Job drawing, mm, ordinate dimensions from the low corner. One solid piece. Round coordinates to 2 decimals unless told otherwise and drop trailing zeros. Order: outer loops, then holes, each group sorted by start corner. A loop starts at its lowest first (then second) coordinate and runs counter-clockwise, first axis right, second up. Notation, with made-up numbers: M 11,78.5 L 64,78.5 A17 cw 64,96.5 Z; hole C 52.5,53 d11. An arc over 180 degrees is marked long. Answer as a JSON object with one key per item and string values. Group by question number.
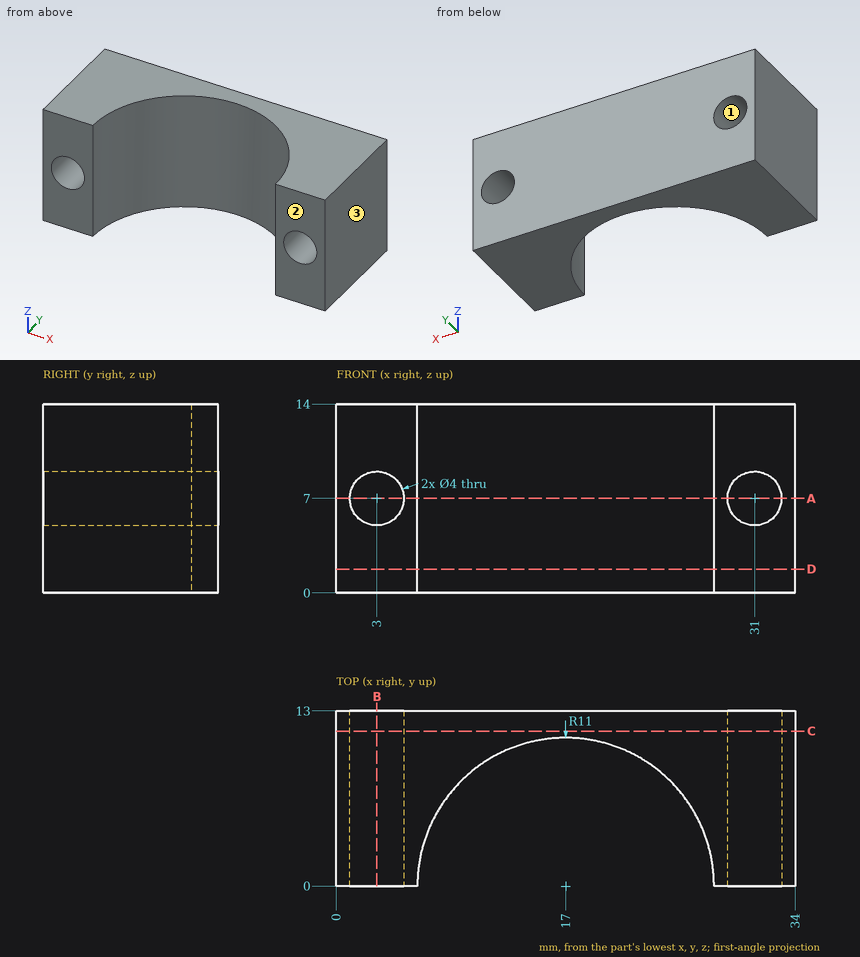
Item 1: Cut at B-B, the plane x = 3. Give the cut face in (y, z), and give its area (3 significant figures).
Item 2: Cut at C-C, the plane y = 11.5. Give the cut face in (x, z), and give its area (3 significant figures).
Item 3: Flat gauge pin, fed straight in: pin 1 Ø1 at (x, z) = (14.5, 12) entering from -Y. Where does the tip first touch, or does it go through?
Item 4: Drill centre lines: line 1 (Z direction, x = 3, y = 2.5); line 2 (X direction, y = 3, z = 7); line 3 (X direction, y = 9, z = 5.5). Where is each one in solid material? Low to high. Write a range as [from, to].
Item 5: Cut at D-D, the plane z = 1.75. Give the cut face in (x, y).
Item 6: Two-plate mould, pull along X, no slides. Class the marked faces 1, 2 and 3: +X half, -X half, draft (parallel to the pull), parting line (faces both ways), or undercut.
Item 7: Cut at A-A, the plane z = 7. Give the cut face in (x, y), and give its area (3 significant figures).
Response values:
{
 "1": {"outline": "M 0,0 L 13,0 L 13,5 L 0,5 Z; M 0,9 L 13,9 L 13,14 L 0,14 Z", "area": "130 mm^2"},
 "2": {"outline": "M 0,0 L 34,0 L 34,14 L 0,14 Z; hole C 3,7 d4; hole C 31,7 d4", "area": "451 mm^2"},
 "3": {"pin 1": "y = 10.58"},
 "4": {"line 1": "[0, 5], [9, 14]", "line 2": "[0, 1], [5, 6.42], [27.58, 29], [33, 34]", "line 3": "[0, 1.68], [4.32, 10.68], [23.32, 29.68], [32.32, 34]"},
 "5": {"outline": "M 0,0 L 6,0 A11 cw 28,0 L 34,0 L 34,13 L 0,13 Z"},
 "6": {"face 1": "undercut", "face 2": "draft", "face 3": "+X half"},
 "7": {"outline": "M 0,0 L 1,0 L 1,13 L 0,13 Z; M 5,0 L 6,0 A11 cw 28,0 L 29,0 L 29,13 L 5,13 Z; M 33,0 L 34,0 L 34,13 L 33,13 Z", "area": "148 mm^2"}
}
